from build123d import *

# Parameters (mm, degrees)
F0_R     = 11.9253
F1_DEPTH = 28.8798
F2_R     = 9.3853
F3_DEPTH = 2.54
F3_TAPER = 60
F4_R     = 9.4996
F5_DEPTH = 16.764
F6_W     = 9.8298
F6_H     = 9.8298
F7_DEPTH = 12.1168001


with BuildPart() as f1:
    # F0 (on Top) → F1 (new body)
    with BuildSketch(Plane.XY):
        Circle(F0_R)
    extrude(amount=F1_DEPTH)

    # F2 (on face) → F3 (cut)
    with BuildSketch(Plane.XY.offset(28.8798)):
        Circle(F2_R)
    extrude(amount=-F3_DEPTH, taper=F3_TAPER, mode=Mode.SUBTRACT)

    # F4 (on face) → F5 (cut)
    with BuildSketch(Plane(origin=(0, 0, 0), x_dir=(1, 0, 0), z_dir=(0, 0, -1))):
        Circle(F4_R)
    extrude(amount=-F5_DEPTH, mode=Mode.SUBTRACT)

    # F6 (on face) → F7 (cut, through all)
    with BuildSketch(Plane(origin=(0, 0, 16.764), x_dir=(1, 0, 0), z_dir=(0, 0, -1))):
        Rectangle(F6_W, F6_H)
    extrude(amount=-F7_DEPTH, mode=Mode.SUBTRACT)


solid = f1.part
Here's how the part is built. I have some questions about the finished solid (model axes, mm). A direction names the side the tool comes from. Give positions to 0.01 mm unless a question says otherwise; leave off trailing zeros. Write each loop counter-clockwise with the first axis right and the second up, starting at its lowest first coordinate (ties: lowest second). Pieces come first, ordered by that corner, then holes. Notation, with made-up numbers: (83, 50) -> (142, 50) arc R16 cw to (142, 59) -> close; hole circle Ø5 at (61.5, -7.5). An arc over 180 degrees is marked (long way). Use one line per item in the form item = value. Start each with the question number.
1. Imagine slicing it at A-A on x = 0. List the corners of the cut face in (y, z) for me, plus the area to 3 significant figures.
2. Imagine slicing it at D-D on z = 13.5. List the corners of the cut face in (x, y) for me.
3. Thinking about a two-plate mould opening in Y: for faces 1 (the face through (6.411, 10.055, 14.238)), 2 (the face through (-1, -10, 0)), 3 (the face through (0, -4.915, 22)), which applies, +Y half, -Y half, draft (parallel to the pull), parting line (faces both ways), or undercut?
4. Will these pins go through, and if not, where does the flat tip stop? pin 1 Ø8 at (y, z) = (6.5, 4.5) entering from +X; pin 2 Ø2 at (y, z) = (7, 4) entering from -X; pin 3 Ø10 at (x, z) = (7.5, 7) entering from +Y.
5. On a 3-axis mill with a long thin cutter (end or side, diameter ignored), from which of +Z, -Z, +X, -X, +Y, -Y can I reach the whole of each face in a straight line? I mean faces 4 (the face through (0, -10, 28.88)), 5 (the face through (4.915, 0, 22)), 6 (the face through (6, 0, 16.764)). Say none if no direction works.
6. If I drill on L1, parallel to Y at x = 0, z = 5.25; L2, parallel to X at y = 0.25, z = 9.5; L3, parallel to Y at x = 0, z = 20.75, over which ranges is the centre line in solid material (lowest first)?
7. Imagine slicing it at B-B on z = 21.5. List the corners of the cut face in (x, y) for me.
8. Imagine slicing it at C-C on x = -10.5. List the corners of the cut face in (y, z) for me, plus the area to 3 significant figures.
Entries:
q1.outline = (-11.93, 0) -> (-9.5, 0) -> (-9.5, 16.76) -> (-4.91, 16.76) -> (-4.91, 26.34) -> (-4.99, 26.34) -> (-9.39, 28.88) -> (-11.93, 28.88) -> close; (4.91, 16.76) -> (9.5, 16.76) -> (9.5, 0) -> (11.93, 0) -> (11.93, 28.88) -> (9.39, 28.88) -> (4.99, 26.34) -> (4.91, 26.34) -> close
q1.area = 240 mm²
q2.outline = circle Ø23.85 at (0, 0); hole circle Ø19 at (0, 0)
q3.face_1 = parting line
q3.face_2 = draft
q3.face_3 = undercut
q4.pin_1 = 11.66
q4.pin_2 = -10.31
q4.pin_3 = 11.66
q5.face_4 = +Z, +X, -X, +Y, -Y
q5.face_5 = +Z, -Z
q5.face_6 = -Z
q6.L1 = -11.93 to -9.5, 9.5 to 11.93
q6.L2 = -11.92 to -9.5, 9.5 to 11.92
q6.L3 = -11.93 to -4.91, 4.91 to 11.93
q7.outline = circle Ø23.85 at (0, 0); hole (-4.91, -4.91) -> (4.91, -4.91) -> (4.91, 4.91) -> (-4.91, 4.91) -> close
q8.outline = (-5.65, 0) -> (5.65, 0) -> (5.65, 28.88) -> (-5.65, 28.88) -> close
q8.area = 327 mm²
